Input: part model. Units: mm. Frame: model coordinates. Face numbers are marked on the shaded views. A direction names the side the tool comes from. Coordinates: 2 decimals unless noted, no trailing zeros. Loops run counter-clockwise (first coordinate to the right, second up) from the corner with the lowest first, then second, coordinate; pieces in that order, holes last. Notation, with made-up numbers: (16, 42.5) -> (43, 42.5) arc R24 cw to (43, 72.5) -> close; hole circle Ø10 at (-29.5, 39). An arc over 180 degrees is marked (long way). Put each result on its own line as item: value. Start each with the question number.
1) Cut plane D-D (z = 12). Return the cut outline in (x, y), plus the area to 3 significant figures.
2) Material intervals for L1, parallel to X at y = 32, z = 60; L2, parallel to X at y = 11, z = 60; L3, parallel to Y at x = -19, z = 41, sorted ascending.
3) Cut plane C-C (y = 10.5). Return the cut outline in (x, z).
4) Set-up query: the marked faces 4, 5, 6 and 7. Return all of +Z, -Z, +X, -X, +Y, -Y with unobstructed straight access to the full face (end or side cutting, diameter ignored); none if empty.
5) Contact query for flat-ended pins moving along their axis: P1, Ø10, axis at y = 34, z = 61, coming from the -X side; P2, Ø6, axis at y = 56.5, z = 8.5, coming from the -X side; P3, Ø13.5, axis at x = -66, z = 16, coming from the +Y side. Output: stop coordinate, or through.
6) Pull-direction query (Z, two-part tool) for the marked faces 1, 2 and 3; classes: pulls with the +Z half, pulls with the -Z half, needs draft (parallel to the pull), parting line crosses it, or undercut.
7) Cut plane B-B (z = 68). Return the cut outline in (x, y).
8) Cut plane A-A (x = -6). Return the cut outline in (y, z), plus the area to 3 significant figures.
from build123d import *

# Parameters (mm, degrees)
SALIENTE_EXTRUIR1_DEPTH    = 80
CROQUIS2_W                 = 30
CROQUIS2_H                 = 20
CORTAR_EXTRUIR1_DEPTH      = 81
CORTAR_EXTRUIR1_DEPTH_BACK = 1
CROQUIS3_W                 = 60
CROQUIS3_H                 = 40
SALIENTE_EXTRUIR2_DEPTH    = 80
CROQUIS4_R                 = 10
CORTAR_EXTRUIR2_DEPTH      = 40


with BuildPart() as part:
    # Croquis1 → Saliente-Extruir1 (new body, symmetric)
    with BuildSketch(Plane(origin=(0, 0, 0), x_dir=(0, 0, -1), z_dir=(1, 0, 0))):
        with BuildLine():
            Line((0, 0), (0, 70))
            Line((0, 70), (-20, 70))
            ThreePointArc((-20, 70), (-40.94875162, 34.138501945), (-80, 20))
            Line((-80, 20), (-80, 0))
            Line((-80, 0), (0, 0))
        make_face()
    extrude(amount=SALIENTE_EXTRUIR1_DEPTH, both=True)

    # Croquis2 → Cortar-Extruir1 (cut, two sides)
    with BuildSketch(Plane.XY) as cortar_extruir1_sk:
        with Locations((-65, 60)):
            Rectangle(CROQUIS2_W, CROQUIS2_H)
        with Locations((65, 60)):
            Rectangle(CROQUIS2_W, CROQUIS2_H)
    extrude(amount=CORTAR_EXTRUIR1_DEPTH, mode=Mode.SUBTRACT)
    extrude(cortar_extruir1_sk.sketch, amount=-CORTAR_EXTRUIR1_DEPTH_BACK, mode=Mode.SUBTRACT)

    # Croquis3 → Saliente-Extruir2 (add)
    with BuildSketch(Plane.XY):
        with Locations((0, 20)):
            Rectangle(CROQUIS3_W, CROQUIS3_H)
    extrude(amount=SALIENTE_EXTRUIR2_DEPTH)

    # Croquis4 → Cortar-Extruir2 (cut)
    with BuildSketch(Plane(origin=(0, 0, 0), x_dir=(1, 0, 0), z_dir=(0, 1, 0))):
        with Locations(Location((0, -60, 0), (0, 0, 270))):  # turned: the seam where the file's is
            Circle(CROQUIS4_R)
    extrude(amount=CORTAR_EXTRUIR2_DEPTH, mode=Mode.SUBTRACT)


solid = part.part
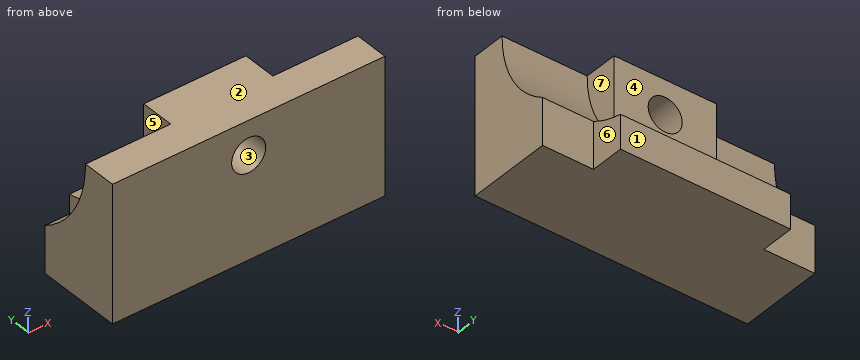
Results found:
1. outline: (-80, 0) -> (80, 0) -> (80, 50) -> (50, 50) -> (50, 70) -> (-50, 70) -> (-50, 50) -> (-80, 50) -> close
1. area: 10,000 mm2
2. L1: x = -30 to -10, 10 to 30
2. L2: x = -80 to -10, 10 to 80
2. L3: y = 0 to 40
3. outline: (-80, 0) -> (80, 0) -> (80, 80) -> (-80, 80) -> close; hole circle Ø20 at (0, 60)
4. face 4: +Z, +X, -X, +Y
4. face 5: +Z, -X, +Y
4. face 6: +Z, -Z, +X, +Y
4. face 7: +Z, +X, +Y
5. P1: stops at x = -30
5. P2: stops at x = -50
5. P3: stops at y = 50
6. face 1: needs draft
6. face 2: pulls with the +Z half
6. face 3: undercut
7. outline: (-80, 0) -> (-6, 0) -> (-6, 40) -> (-30, 40) -> (-30, 21.19) -> (-80, 21.19) -> close; (6, 0) -> (80, 0) -> (80, 21.19) -> (30, 21.19) -> (30, 40) -> (6, 40) -> close
8. outline: (0, 0) -> (70, 0) -> (70, 20) arc R61 cw to (40, 34.83) -> (40, 52) -> (0, 52) -> close; (0, 68) -> (40, 68) -> (40, 80) -> (0, 80) -> close
8. area: 3,330 mm2
